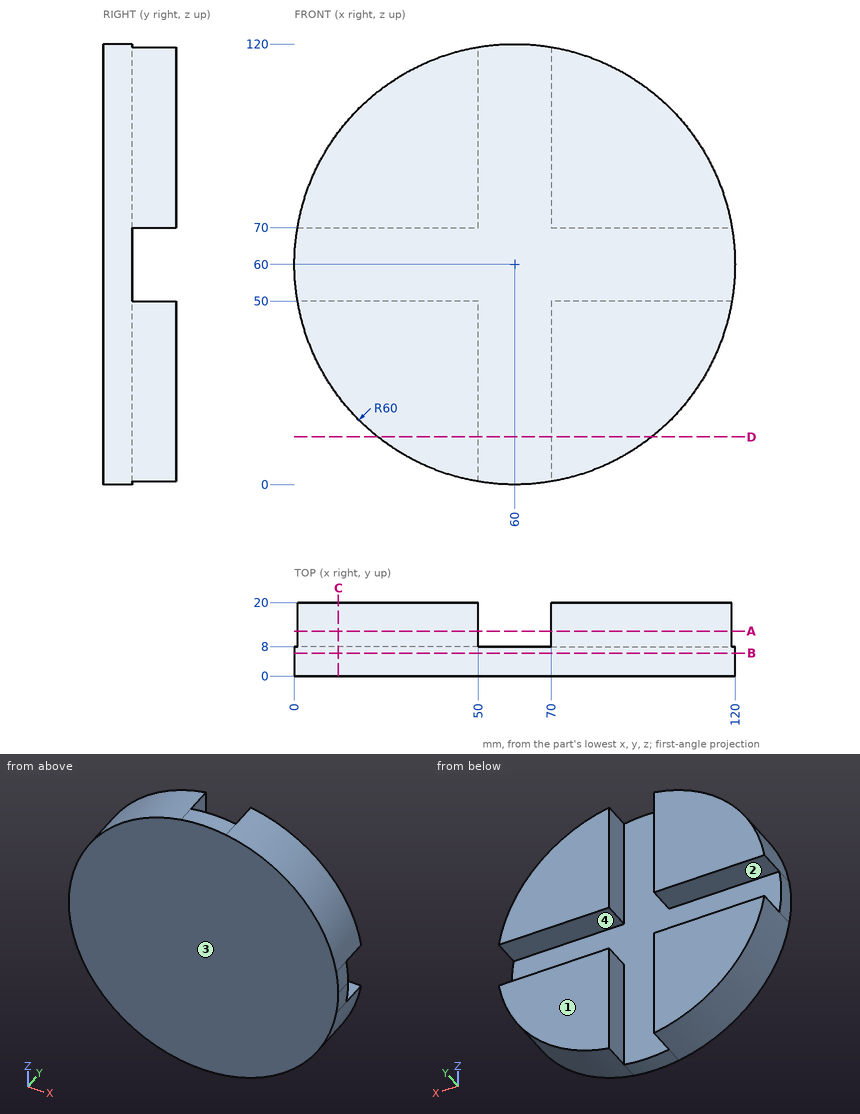
Study the drawing (mm; zero at the part's minimum x, y, z) and answer. A direction names the side the tool comes from. Give positions to 0.01 mm unless a question says otherwise; leave off trailing zeros. Write each loop counter-clockwise with the first axis right and the second up, starting at its lowest first coordinate (ties: lowest second). Pieces come first, ordered by that corner, then holes. Notation, with made-up numbers: (-33.75, 8) -> (9.25, 8) arc R23 ccw to (9.25, 38) -> close; hole circle Ø1 at (-12.5, 53.25). An arc over 180 degrees is marked (long way). Write item = value, one per line. Start each with the question number.
1) The part is cut by section D-D, the plane z = 13. Determine the outline of the cut face in (x, y).
2) The part is cut by section B-B, the plane y = 6.25. Determine the outline of the cut face in (x, z), and give its area (3 significant figures).
3) Which of the six approach directions +Z, -Z, +X, -X, +Y, -Y give full straight-line access (tool end or side, diameter ignored) to the marked faces 3 and 4?
4) Straight lines are drawn through the part: line 1 along Y through (x, z) = (59, 29.5); line 2 along Z through (x, y) = (114, 16.5); line 3 along Z through (x, y) = (26.5, 17.5). For each, find the intervals that lie inside material, in ascending order.
5) Determine the mould class of the marked faces 1 and 2 for opening direction Z: +Z half, -Z half, draft (parallel to the pull), parting line (faces both ways), or undercut.
6) The part is cut by section A-A, the plane y = 12.25. Determine the outline of the cut face in (x, z).
7) The part is cut by section C-C, the plane x = 12. Determine the outline of the cut face in (y, z), and give its area (3 significant figures).
8) Each of these flat-tipped pins is pushed along its axis until it touches: pin 1 (9.5 mm diameter, centred on x = 83, y = 11.5, fed in from -Z); pin 2 (3 mm diameter, centred on y = 11.5, z = 46.5, fed in from +X); pin 3 (5 mm diameter, centred on x = 97, y = 16.5, fed in from -Z). Where does it stop, or does it pass through?
Solutions:
q1.outline = (22.7, 0) -> (97.3, 0) -> (97.3, 20) -> (70, 20) -> (70, 8) -> (50, 8) -> (50, 20) -> (22.7, 20) -> close
q2.outline = circle Ø120 at (60, 60)
q2.area = 11,300 mm²
q3.face_3 = +Z, -Z, +X, -X, -Y
q3.face_4 = +X, -X, +Y
q4.line_1 = 0 to 8
q4.line_2 = 33.85 to 50, 70 to 86.15
q4.line_3 = 10.22 to 50, 70 to 109.78
q5.face_1 = draft
q5.face_2 = undercut
q6.outline = (0.84, 50) arc R60 ccw to (50, 0.84) -> (50, 50) -> close; (0.84, 70) -> (50, 70) -> (50, 119.16) arc R60 ccw to start; (70, 0.84) arc R60 ccw to (119.16, 50) -> (70, 50) -> close; (70, 70) -> (119.16, 70) arc R60 ccw to (70, 119.16) -> close
q7.outline = (0, 24) -> (20, 24) -> (20, 50) -> (8, 50) -> (8, 70) -> (20, 70) -> (20, 96) -> (0, 96) -> close
q7.area = 1,200 mm²
q8.pin_1 = 2.84
q8.pin_2 = 118.79
q8.pin_3 = 10.91
